```python
from build123d import *

# Parameters (mm, degrees)
F0_W     = 121
F0_H     = 16
F1_DEPTH = 57
F3_DEPTH = 33
F5_DEPTH = 33
F6_R     = 7
F7_DEPTH = 16.001


with BuildPart() as f1:
    # F0 (on Top) → F1 (new body)
    with BuildSketch(Plane.XY):
        with Locations((60.5, 8)):
            Rectangle(F0_W, F0_H)
    extrude(amount=F1_DEPTH)

    # F2 (on face) → F3 (join)
    with BuildSketch(Plane.XZ):
        Polygon((18.79299, 25.615024), (0, 46), (0, 0), (18.79299, 0), align=None)
        Polygon((42.407583, 0), (18.79299, 25.615024), (18.79299, 0), align=None)
    extrude(amount=F3_DEPTH)

    # F4 (on face) → F5 (join)
    with BuildSketch(Plane.XZ):
        Polygon((121, 11), (121, 57), (60.5, 57), align=None)
    extrude(amount=F5_DEPTH)

    # F6 (on face) → F7 (cut, through all)
    with BuildSketch(Plane.XZ):
        with Locations((28.861878, 41.622804)):
            Circle(F6_R)
        with Locations((68.02547, 15.911056)):
            Circle(F6_R)
    extrude(amount=-F7_DEPTH, mode=Mode.SUBTRACT)


solid = f1.part
```
Here's how the part is built. I have some questions about the finished solid (model axes, mm). A direction names the side the tool comes from. Give positions to 0.01 mm unless a question says otherwise; leave off trailing zeros. Write each loop counter-clockwise with the first axis right and the second up, starting at its lowest first coordinate (ties: lowest second). Pieces come first, ordered by that corner, then holes. Notation, with made-up numbers: (85.5, 8.5) -> (122.5, 8.5) arc R17 cw to (122.5, 29.5) -> close; hole circle Ø11 at (-21.5, -40). An arc over 180 degrees is marked (long way). Write each question's results on one line, items separated by ' | '.
Item 1: Suppose I cut it at D-D on y = 7. Write out the boundary of the cut face in (x, z), plus the area to 3 significant figures.
Output:
outline: (0, 0) -> (121, 0) -> (121, 57) -> (0, 57) -> close; hole circle Ø14 at (28.86, 41.62); hole circle Ø14 at (68.03, 15.91) | area: 6,590 mm^2
Item 2: Suppose I cut it at C-C on x = 47.5. Write out the boundary of the cut face in (y, z), plus the area to 3 significant figures.
Output:
outline: (0, 0) -> (16, 0) -> (16, 57) -> (0, 57) -> close | area: 912 mm^2
Item 3: Suppose I cut it at A-A on y = -22. Write out the boundary of the cut face in (x, z).
Output:
outline: (0, 0) -> (42.41, 0) -> (0, 46) -> close; (60.5, 57) -> (121, 11) -> (121, 57) -> close
Item 4: Suppose I cut it at B-B on z = 44.5. Write out the boundary of the cut face in (x, y).
Output:
outline: (0, -33) -> (1.38, -33) -> (1.38, 0) -> (22.48, 0) -> (22.48, 16) -> (0, 16) -> close; (35.24, 0) -> (76.94, 0) -> (76.94, -33) -> (121, -33) -> (121, 16) -> (35.24, 16) -> close
Item 5: We'd pull the mould along Z, two halves only. Please class faces 1 (the face through (27.3, 7.9, 34.8)), 2 (the face through (90.33, -16.27, 34.32)), 3 (the face through (74.702, 7.888, 18.014)), 4 (the face through (75, -3, 57)): pulls with the +Z half, pulls with the -Z half, needs draft (parallel to the pull), parting line crosses it, or undercut.
Output:
face 1: undercut | face 2: pulls with the -Z half | face 3: undercut | face 4: pulls with the +Z half
Item 6: If I drill on L1, parallel to X at y = 0.5, z = 16; L2, parallel to Y at x = 44.5, z = 41; L3, parallel to X at y = -16, z = 14, over which ranges is the centre line in solid material (lowest first)?
Output:
L1: x = 0 to 61.03, 75.02 to 121 | L2: y = 0 to 16 | L3: x = 0 to 29.5, 117.05 to 121
Item 7: On a 3-axis mill with a long thin cutter (end or side, diameter ignored), from which of +Z, -Z, +X, -X, +Y, -Y can I reach the whole of each face in a straight line? I mean faces 5 (the face through (60, 0, 28)), 6 (the face through (60, 16, 28)). Say none if no direction works.
Output:
face 5: -Y | face 6: +Z, -Z, +X, -X, +Y
Item 8: For pin 1 Ø6 at (x, z) = (78, 10) entering from -Y; pin 2 Ø4 at (x, y) = (57, -6.5) entering from -Z, each with a flat end and sliding along its axis, tell me the tip position at first contact or that it passes through.
Output:
pin 1: stops at y = 0 | pin 2: passes through
